```python
from build123d import *

# Parameters (mm, degrees)
F1_DEPTH = 50.8
F2_R     = 851.2175
F3_DEPTH = 50.8
F4_W     = 254
F4_H     = 762
F4_R     = 50.8
F5_DEPTH = 857.5685
F7_R     = 6.35


with BuildPart() as f1:
    # F0 (on Right) → F1 (new body, symmetric)
    with BuildSketch(Plane.YZ):
        with BuildLine():
            Line((-794.0675, -323.85), (-794.0675, 323.85))
            ThreePointArc((-794.0675, 323.85), (-857.5675, 0), (-794.0675, -323.85))
        make_face()
    extrude(amount=F1_DEPTH, both=True)

    # F2 (on Right) → F3 (cut, symmetric)
    with BuildSketch(Plane.YZ):
        Circle(F2_R)
    extrude(amount=F3_DEPTH, both=True, mode=Mode.SUBTRACT)

    # F4 (on Front) → F5 (cut, through all)
    with BuildSketch(Plane.XZ):
        Rectangle(F4_W, F4_H)
        with Locations((0, 196.85)):
            Circle(F4_R, mode=Mode.SUBTRACT)
    extrude(amount=F5_DEPTH, mode=Mode.SUBTRACT)

    # F7 (on offset) → F8 (join, up to the next surface of F1)
    with BuildSketch(Plane.XZ.offset(787.4)):
        with Locations((38.1, 196.85)):
            Circle(F7_R)
    extrude(until=Until.NEXT)


solid = f1.part
```
Source: CAD feature listing. Evaluate the final solid. Frame: model axes, mm. A direction names the side the tool comes from. Round coordinates to 2 decimals unless told otherwise and drop trailing zeros. Loops run counter-clockwise (first coordinate to the right, second up) from the corner with the lowest first, then second, coordinate; pieces in that order, holes last. Notation, with made-up numbers: M 68,-7.5 L 92,-7.5 A10 ccw 92,11.5 Z; hole C 75,2.5 d7. An arc over 180 degrees is marked long. Put each result on its own line as item: value.
(1) Section B-B, the plane z = 196.85. Return loops of the section in (x, y), and give its area (3 significant figures).
Solutions:
outline: M -50.8,-834.67 L 50.8,-834.67 L 50.8,-828.14 L 44.45,-828.14 L 44.45,-787.4 L 31.75,-787.4 L 31.75,-828.14 L -50.8,-828.14 Z
area: 1,180 mm²
(2) Access query for faces 1 (the face through (36.72, -808.22, 190.65)), 2 (the face through (0.701, -834.414, 197.927)). Directions: +Z, -Z, +X, -X, +Y, -Y. A direction counts if a zero-diameter tool reaches every point of the face in a straight line with its end or side. Return the directions, or none.
Solutions:
face 1: +Y
face 2: +Z, +X, -X, -Y
(3) Section D-D, the plane y = -809. Return loops of the section in (x, z), and give its area (3 significant figures).
Solutions:
outline: C 38.1,196.85 d12.7
area: 127 mm²
(4) First-contact query: pin 1 (5 mm diameter, centred on x = 2, z = 225, fed in from +Y); pin 2 (8 mm diameter, centred on y = -795.5, z = 183, fed in from +X); pin 3 (1 mm diameter, centred on x = -17, y = -817, fed in from +Z); pin 4 (4 mm diameter, centred on x = -9, z = 183, fed in from +Y). Flat tips, straight axial feed; report the tip coordinate or a pass-through.
Solutions:
pin 1: y = -820.25
pin 2: through
pin 3: z = 244.9
pin 4: y = -830.87
(5) Ray query, line 1 (Y direction, x = -2, z = 198); line 2 (Y direction, x = -6, z = 189.5); line 3 (Z direction, x = 41, y = -806). Return the intervals inside material, ascending. Write a range as [from, to].
Solutions:
line 1: [-834.4, -827.87]
line 2: [-836.37, -829.86]
line 3: [191.2, 202.5]
(6) Section C-C, the plane y = -824. Return loops of the section in (x, z), and give its area (3 significant figures).
Solutions:
outline: M -47.98,213.53 L 47.98,213.53 A50.8 ccw 30.35,237.58 L -30.35,237.58 A50.8 ccw Z; C 38.1,196.85 d12.7
area: 2,100 mm²
(7) Section A-A, the plane x = 38.1. Return loops of the section in (y, z) (1 decimal), and give its area (3 significant figures).
Solutions:
outline: M -841.9,163.2 L -835.4,163.2 A851.2 cw -829.6,190.5 L -787.4,190.5 L -787.4,203.2 L -826.6,203.2 A851.2 cw -819.4,230.5 L -826,230.5 A857.6 ccw Z
area: 956 mm²
